Read the model definition and answer for the solid it produces. Units are mm, in the model's axes. A direction names the side the tool comes from. Coordinates: 2 decimals unless noted, no trailing zeros. Order: outer loops, then holes, each group sorted by start corner. A loop starts at its lowest first (then second) coordinate and runs counter-clockwise, first axis right, second up.
from build123d import *

# Parameters (mm, degrees)
CROQUIS1_W                   = 12.5
CROQUIS1_H                   = 5.9
CROQUIS1_W_2                 = 0.64
CROQUIS1_H_2                 = 0.8
SALIENTE_EXTRUIR1_DEPTH      = 1
CROQUIS2_W                   = 12.5
CROQUIS2_H                   = 5.9
CROQUIS2_W_2                 = 11
CROQUIS2_H_2                 = 4.4
SALIENTE_EXTRUIR2_DEPTH      = 6
CORTAR_EXTRUIR1_DEPTH        = 9
CORTAR_EXTRUIR2_DEPTH        = 2
SALIENTE_EXTRUIR3_DEPTH      = 6.5
SALIENTE_EXTRUIR3_DEPTH_BACK = 3.4
CROQUIS5_W                   = 0.64
CROQUIS5_H                   = 0.8


with BuildPart() as part:
    # Croquis1 → Saliente-Extruir1 (new body)
    with BuildSketch(Plane(origin=(0, 0, 0), x_dir=(1, 0, 0), z_dir=(0, 1, 0))):
        with Locations((3.77, 0.42)):
            Rectangle(CROQUIS1_W, CROQUIS1_H)
        Rectangle(CROQUIS1_W_2, CROQUIS1_H_2, mode=Mode.SUBTRACT)
        with Locations((7.54, 0)):
            Rectangle(CROQUIS1_W_2, CROQUIS1_H_2, mode=Mode.SUBTRACT)
        with Locations((5.04, 0)):
            Rectangle(CROQUIS1_W_2, CROQUIS1_H_2, mode=Mode.SUBTRACT)
        with Locations((2.5, 0)):
            Rectangle(CROQUIS1_W_2, CROQUIS1_H_2, mode=Mode.SUBTRACT)
    extrude(amount=SALIENTE_EXTRUIR1_DEPTH)

    # Croquis2 → Saliente-Extruir2 (add)
    with BuildSketch(Plane(origin=(0, 1, 0), x_dir=(1, 0, 0), z_dir=(0, 1, 0))):
        with Locations((3.77, 0.42)):
            Rectangle(CROQUIS2_W, CROQUIS2_H)
        with Locations((3.77, 0.42)):
            Rectangle(CROQUIS2_W_2, CROQUIS2_H_2, mode=Mode.SUBTRACT)
    extrude(amount=SALIENTE_EXTRUIR2_DEPTH)

    # Croquis3 → Cortar-Extruir1 (cut)
    with BuildSketch(Plane.ZY.offset(2.48)):
        with BuildLine():
            Line((1.78, 7), (1.78, 4.35))
            ThreePointArc((1.78, 4.35), (1.604264069, 3.925735931), (1.18, 3.75))
            Line((1.18, 3.75), (0.78, 3.75))
            Line((0.78, 3.75), (0.78, 7))
            Line((0.78, 7), (1.78, 7))
        make_face()
    extrude(amount=-CORTAR_EXTRUIR1_DEPTH, mode=Mode.SUBTRACT)

    # Croquis4 → Cortar-Extruir2 (cut)
    with BuildSketch(Plane.XY.offset(2.53)):
        with BuildLine():
            Line((-0.48, 7), (-0.48, 3.85))
            ThreePointArc((-0.48, 3.85), (-0.304264069, 3.425735931), (0.12, 3.25))
            Line((0.12, 3.25), (1.02, 3.25))
            Line((1.02, 3.25), (1.02, 7))
            Line((1.02, 7), (-0.48, 7))
        make_face()
        with BuildLine():
            Line((8.02, 7), (6.52, 7))
            Line((6.52, 7), (6.52, 3.25))
            Line((6.52, 3.25), (7.42, 3.25))
            ThreePointArc((7.42, 3.25), (7.844264069, 3.425735931), (8.02, 3.85))
            Line((8.02, 3.85), (8.02, 7))
        make_face()
    extrude(amount=-CORTAR_EXTRUIR2_DEPTH, mode=Mode.SUBTRACT)

    # Croquis5 → Saliente-Extruir3 (add, two sides: drawn at the far end of the back side and taken through both)
    with BuildSketch(Plane(origin=(0, 0, 0), x_dir=(1, 0, 0), z_dir=(0, 1, 0)).offset(-SALIENTE_EXTRUIR3_DEPTH_BACK)):
        with Locations((7.54, 0)):
            Rectangle(CROQUIS5_W, CROQUIS5_H)
        Rectangle(CROQUIS5_W, CROQUIS5_H)
        with Locations((2.5, 0)):
            Rectangle(CROQUIS5_W, CROQUIS5_H)
        with Locations((5.04, 0)):
            Rectangle(CROQUIS5_W, CROQUIS5_H)
    extrude(amount=SALIENTE_EXTRUIR3_DEPTH + SALIENTE_EXTRUIR3_DEPTH_BACK)


solid = part.part
Q1. The part is cut by section A-A, the plane y = 2.25. Determine the outline of the cut face in (x, z).
Q2. The part is cut by section C-C, the plane x = 0.5. Determine the outline of the cut face in (y, z).
Q3. The part is cut by section D-D, the plane y = -0.25. Determine the outline of the cut face in (x, z), then the cut area to 3 significant figures.
Q4. The part is cut by section B-B, the plane y = 5.75. State how many separate pieces and enclosed holes the cut face has, then the cut area to 3 significant figures.
Q5. Straight lines are drawn through the part: L1, parallel to X at y = -2.25, z = 0; L2, parallel to X at y = 3, z = -0.1; L3, parallel to Z at x = 5, y = 4.25. For each, find the intervals that lie inside material, in ascending order.
Q6. Determine the mould class of faces 3 (the flat face through (4, 3, 2.53)), 4 (the flat face through (4, 3, -3.37)), 5 (the flat face through (4, 1, 0)), 6 (the flat face through (4, 0, 0)) for opening direction Z: +Z half, -Z half, draft (parallel to the pull), parting line (faces both ways), or undercut.
Q7. Which of the six approach directions +Z, -Z, +X, -X, +Y, -Y give full straight-line access (tool end or side, diameter ignored) to faces 1 (the flat face through (-1.73, 4, 0)), 2 (the flat face through (4, 7, -3))?
Q8. Each of these flat-tipped pins is pushed along its axis until it touches: P1, Ø1.5, axis at x = 1.5, y = -1.5, coming from the +Z side; P2, Ø0.6, axis at y = -2, z = 0, coming from the -X side; P3, Ø0.6, axis at x = 0.5, z = 2.5, coming from the +Y side. Where does it stop, or does it pass through?
Computed values:
1. outline: (-2.48, -3.37) - (10.02, -3.37) - (10.02, 2.53) - (-2.48, 2.53) - close; (-0.32, -0.4) - (0.32, -0.4) - (0.32, 0.4) - (-0.32, 0.4) - close; (2.18, -0.4) - (2.82, -0.4) - (2.82, 0.4) - (2.18, 0.4) - close; (4.72, -0.4) - (5.36, -0.4) - (5.36, 0.4) - (4.72, 0.4) - close; (7.22, -0.4) - (7.86, -0.4) - (7.86, 0.4) - (7.22, 0.4) - close; hole (-1.73, -2.62) - (9.27, -2.62) - (9.27, 1.78) - (-1.73, 1.78) - close
2. outline: (0, -3.37) - (7, -3.37) - (7, -2.62) - (1, -2.62) - (1, 1.78) - (3.25, 1.78) - (3.25, 2.53) - (0, 2.53) - close
3. outline: (-0.32, -0.4) - (0.32, -0.4) - (0.32, 0.4) - (-0.32, 0.4) - close; (2.18, -0.4) - (2.82, -0.4) - (2.82, 0.4) - (2.18, 0.4) - close; (4.72, -0.4) - (5.36, -0.4) - (5.36, 0.4) - (4.72, 0.4) - close; (7.22, -0.4) - (7.86, -0.4) - (7.86, 0.4) - (7.22, 0.4) - close
3. area: 2.05 mm2
4. separate pieces: 7
4. enclosed holes: 0
4. area: 24.4 mm2
5. L1: x = -0.32 to 0.32, 2.18 to 2.82, 4.72 to 5.36, 7.22 to 7.86
5. L2: x = -2.48 to -1.73, -0.32 to 0.32, 2.18 to 2.82, 4.72 to 5.36, 7.22 to 7.86, 9.27 to 10.02
5. L3: z = -3.37 to -2.62, -0.4 to 0.4, 1.78 to 2.53
6. face 3: +Z half
6. face 4: -Z half
6. face 5: undercut
6. face 6: draft
7. face 1: +Y
7. face 2: +Z, -Z, +X, -X, +Y
8. P1: stops at z = 0.4
8. P2: stops at x = -0.32
8. P3: stops at y = 3.25
